Print and shaded views of the part. All mm, measured from the part's lowest x, y and z. A direction names the side the tool comes from. Round coordinates to 2 decimals unless told otherwise and drop trailing zeros. Order: outer loops, then holes, each group sorted by start corner. A loop starts at its lowest first (then second) coordinate and runs counter-clockwise, first axis right, second up.
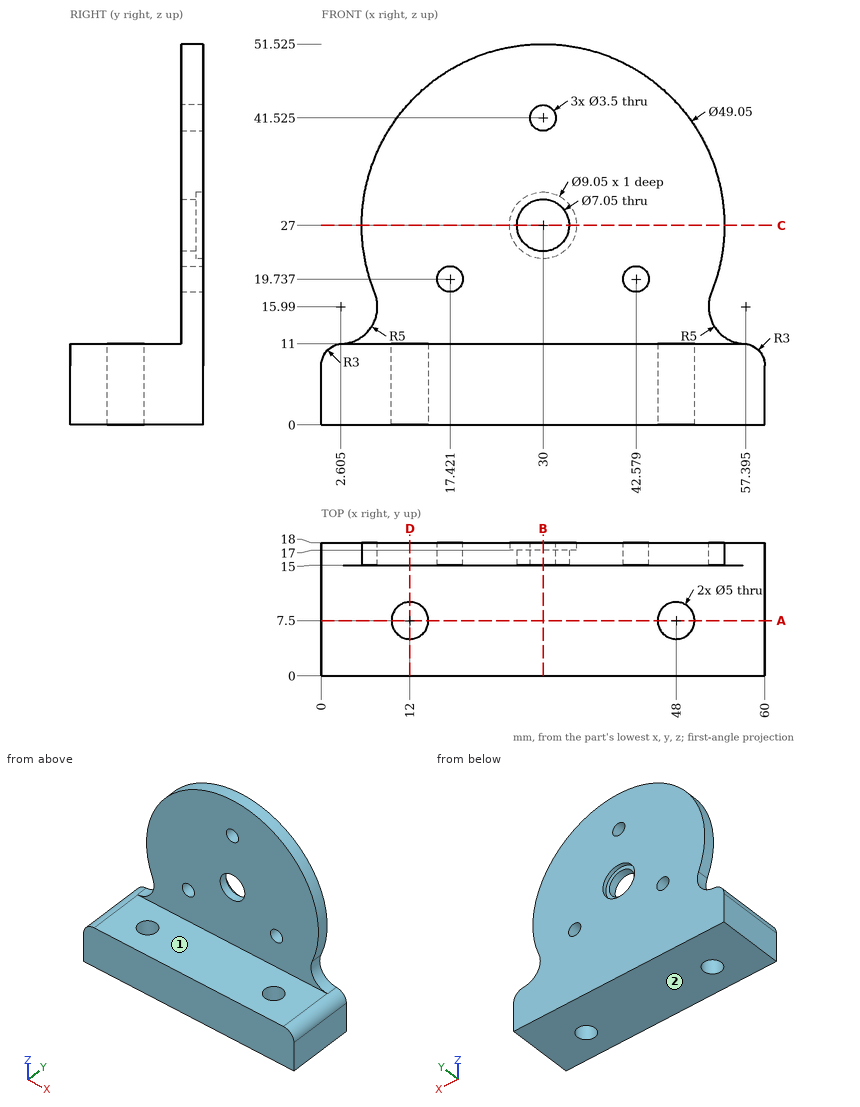
1. Cut at C-C, the plane z = 27. Write the cut outline in (x, y) (1 decimal).
2. Tool access for the marked faces 1 and 2: list every direction of +Z, -Z, +X, -X, +Y, -Y with a clear straight run to the whole face (end or side of a thin tool).
3. Cut at D-D, the plane x = 12. Write the cut outline in (y, z), and give its area (3 significant figures).
4. Cut at B-B, the plane x = 30. Write the cut outline in (y, z) (1 decimal), and give its area (3 significant figures).
5. Drill centre lines: line 1 (X direction, y = 6.5, z = 9.5); line 2 (X direction, y = 17.3, z = 27) (1 decimal); line 3 (X direction, y = 6.5, z = 6). Where is each one in solid material? Low to high.
6. Cut at A-A, the plane y = 7.5. Write the cut outline in (x, z).
7. Pin check, flat tips, straight feed: P1, Ø5, axis at x = 46, y = 4.5, coming from the +Z side; P2, Ø6, axis at y = 12, z = 6, coming from the -X side; P3, Ø14.5, axis at x = 30, z = 27, coming from the -Y side; P4, Ø2, axis at x = 30, z = 41.525, coming from the +Y side. Stop position of each tip, or through.
Outcome:
1. outline: (5.5, 15) - (26.5, 15) - (26.5, 17) - (25.5, 17) - (25.5, 18) - (5.5, 18) - close; (33.5, 15) - (54.5, 15) - (54.5, 18) - (34.5, 18) - (34.5, 17) - (33.5, 17) - close
2. face 1: +Z, +X, -X, -Y
2. face 2: -Z, +X, -X, +Y, -Y
3. outline: (0, 0) - (5, 0) - (5, 11) - (0, 11) - close; (10, 0) - (18, 0) - (18, 43.66) - (15, 43.66) - (15, 11) - (10, 11) - close
3. area: 241 mm2
4. outline: (0, 0) - (18, 0) - (18, 22.5) - (17, 22.5) - (17, 23.5) - (15, 23.5) - (15, 11) - (0, 11) - close; (15, 30.5) - (17, 30.5) - (17, 31.5) - (18, 31.5) - (18, 39.8) - (15, 39.8) - close; (15, 43.3) - (18, 43.3) - (18, 51.5) - (15, 51.5) - close
4. area: 286 mm2
5. line 1: x = 0.4 to 9.71, 14.29 to 45.71, 50.29 to 59.6
5. line 2: x = 5.5 to 25.5, 34.5 to 54.5
5. line 3: x = 0 to 9.71, 14.29 to 45.71, 50.29 to 60
6. outline: (0, 0) - (9.5, 0) - (9.5, 11) - (3, 11) arc R3 ccw to (0, 8) - close; (14.5, 0) - (45.5, 0) - (45.5, 11) - (14.5, 11) - close; (50.5, 0) - (60, 0) - (60, 8) arc R3 ccw to (57, 11) - (50.5, 11) - close
7. P1: stops at z = 11
7. P2: stops at x = 0
7. P3: stops at y = 15
7. P4: passes through
